Source: CAD feature listing. Evaluate the final solid. Frame: model axes, mm. Face numbers are marked on the shaded views. A direction names the side the tool comes from. Round coordinates to 2 decimals unless told otherwise and drop trailing zeros. Loops run counter-clockwise (first coordinate to the right, second up) from the corner with the lowest first, then second, coordinate; pieces in that order, holes last. Notation, with made-up numbers: M 76.25,-5 L 134.25,-5 A22 ccw 134.25,12 Z; hole C -33,-23 d4. An arc over 180 degrees is marked long. One line per item, written item: value.
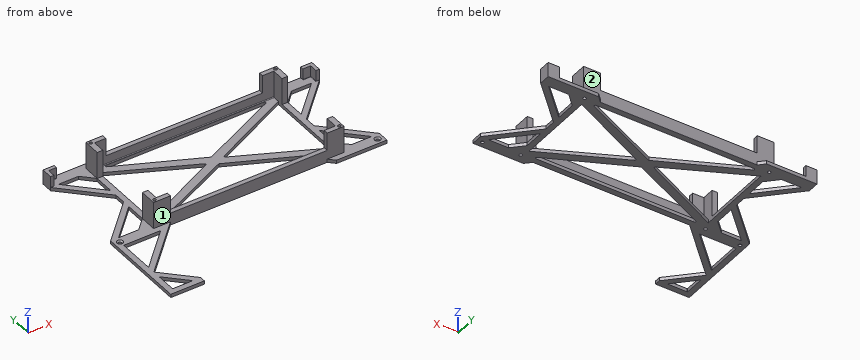
from build123d import *

# Parameters (mm, degrees)
SKETCH003_W     = 170
SKETCH003_H     = 90
SKETCH003_W_2   = 160
SKETCH003_H_2   = 80
PAD_DEPTH       = 3
PAD001_DEPTH    = 3
PAD002_DEPTH    = 3
PAD003_DEPTH    = 3
PAD004_DEPTH    = 3
PAD005_DEPTH    = 10
PAD006_DEPTH    = 10
PAD007_DEPTH    = 24
SKETCH014_R     = 1.65
HOLE_DEPTH      = 30
SKETCH015_R     = 1.325
HOLE001_DEPTH   = 30
SKETCH016_R     = 1.325
HOLE002_DEPTH   = 30
SKETCH017_R     = 1.325
HOLE003_DEPTH   = 30
FILLET_R        = 0.3
FILLET001_R     = 0.3
FILLET002_R     = 0.3
FILLET003_R     = 0.3
FILLET004_R     = 0.3
FILLET005_R     = 0.3
FILLET006_R     = 0.3
FILLET007_R     = 0.3
FILLET008_R     = 0.3
FILLET009_R     = 0.3
SKETCH018_W     = 3.707428
SKETCH018_H     = 3.707435
PAD008_DEPTH    = 27
SKETCH019_W     = 4.325348
SKETCH019_H     = 3.769226
PAD009_DEPTH    = 27
SKETCH020_W     = 4.473305
SKETCH020_H     = 4.349049
PAD010_DEPTH    = 27
SKETCH021_W     = 3.413819
SKETCH021_H     = 3.638272
PAD011_DEPTH    = 27
SKETCH023_R     = 1.4
POCKET_DEPTH    = 30
SKETCH024_R     = 1.4
POCKET001_DEPTH = 30
SKETCH025_R     = 1.4
POCKET002_DEPTH = 30
SKETCH026_R     = 1.4
POCKET003_DEPTH = 30
SKETCH027_R     = 1.5
POCKET004_DEPTH = 5
CHAMFER_SIZE    = 1.2
SKETCH028_W     = 10
SKETCH028_H     = 1
POCKET005_DEPTH = 24
SKETCH029_W     = 10
SKETCH029_H     = 1
POCKET006_DEPTH = 24
SKETCH030_W     = 10
SKETCH030_H     = 1
POCKET007_DEPTH = 24
PAD012_DEPTH    = 3
SKETCH032_W     = 140
SKETCH032_H     = 4
PAD013_DEPTH    = 8
FILLET010_R     = 0.7
FILLET011_R     = 1


with BuildPart() as part:
    # Sketch003 → Pad (new body)
    with BuildSketch(Plane.XY):
        Rectangle(SKETCH003_W, SKETCH003_H)
        Rectangle(SKETCH003_W_2, SKETCH003_H_2, mode=Mode.SUBTRACT)
    extrude(amount=PAD_DEPTH)

    # Sketch005 → Pad001 (join)
    with BuildSketch(Plane.XY):
        Polygon((-70, 45), (-75, 50), (-120, 50), (-120, 40), (-85, 5), (-85, 12), (-113, 40), (-95, 40), (-85, 30), (-85, 45), align=None)
    extrude(amount=PAD001_DEPTH)

    # Sketch007 → Pad002 (join)
    with BuildSketch(Plane.XY):
        Polygon((70, 45), (75, 50), (120, 50), (120, 40), (85, 5), (85, 12), (113, 40), (95, 40), (85, 30), (85, 45), align=None)
    extrude(amount=PAD002_DEPTH)

    # Sketch008 → Pad003 (join)
    with BuildSketch(Plane.XY):
        Polygon((70, -45), (75, -50), (120, -50), (120, -40), (85, -5), (85, -12), (113, -40), (95, -40), (85, -30), (85, -45), align=None)
    extrude(amount=PAD003_DEPTH)

    # Sketch009 → Pad004 (join)
    with BuildSketch(Plane.XY):
        Polygon((-70, -45), (-75, -50), (-115, -90), (-90, -115), (-90, -120), (-120, -120), (-120, -50), (-120, -40), (-85, -5), (-85, -12), (-113, -40), (-95, -40), (-85, -30), (-85, -45), align=None)
        Polygon((-115, -50), (-115, -83), (-82, -50), align=None, mode=Mode.SUBTRACT)
        Polygon((-115, -97), (-115, -115), (-97, -115), align=None, mode=Mode.SUBTRACT)
    extrude(amount=PAD004_DEPTH)

    # Sketch011 (on Face23 of Pad004) → Pad005 (join)
    with BuildSketch(Plane.XY.offset(3)):
        Polygon((-120, 50), (-120, 40), (-117, 40), (-117, 47), (-110, 47), (-110, 50), align=None)
    extrude(amount=PAD005_DEPTH)

    # Sketch012 (on Face22 of Pad005) → Pad006 (join)
    with BuildSketch(Plane.XY.offset(3)):
        Polygon((120, 50), (110, 50), (110, 47), (117, 47), (117, 40), (120, 40), align=None)
    extrude(amount=PAD006_DEPTH)

    # Sketch013 (on Face4 of Pad006) → Pad007 (join)
    with BuildSketch(Plane.XY.offset(3)):
        Polygon((-85, 45), (-85, 30), (-80, 30), (-80, 40), (-70, 40), (-70, 45), align=None)
        Polygon((85, 45), (85, 30), (80, 30), (80, 40), (70, 40), (70, 45), align=None)
        Polygon((85, -45), (85, -30), (80, -30), (80, -40), (70, -40), (70, -45), align=None)
        Polygon((-85, -45), (-85, -30), (-80, -30), (-80, -40), (-70, -40), (-70, -45), align=None)
    extrude(amount=PAD007_DEPTH)

    # Sketch014 (on Face80 of Pad007) → Hole (cut)
    with BuildSketch(Plane.XY.offset(27)):
        with Locations((-82.5, 42.5)):
            Circle(SKETCH014_R)
    extrude(amount=-HOLE_DEPTH, mode=Mode.SUBTRACT)

    # Sketch015 (on Face99 of Hole) → Hole001 (cut)
    with BuildSketch(Plane.XY.offset(27)):
        with Locations((-82.5, -42.5)):
            Circle(SKETCH015_R)
    extrude(amount=-HOLE001_DEPTH, mode=Mode.SUBTRACT)

    # Sketch016 (on Face84 of Hole001) → Hole002 (cut)
    with BuildSketch(Plane.XY.offset(27)):
        with Locations((82.5, 42.5)):
            Circle(SKETCH016_R)
    extrude(amount=-HOLE002_DEPTH, mode=Mode.SUBTRACT)

    # Sketch017 (on Face104 of Hole002) → Hole003 (cut)
    with BuildSketch(Plane.XY.offset(27)):
        with Locations((82.5, -42.5)):
            Circle(SKETCH017_R)
    extrude(amount=-HOLE003_DEPTH, mode=Mode.SUBTRACT)

    # Fillet
    fillet_edges = [part.edges().sort_by_distance(p)[0] for p in [
        (-115, -97, 1.5),
    ]]
    fillet(fillet_edges, radius=FILLET_R)

    # Fillet001
    fillet001_edges = [part.edges().sort_by_distance(p)[0] for p in [
        (-115, -115, 1.5),
    ]]
    fillet(fillet001_edges, radius=FILLET001_R)

    # Fillet002
    fillet002_edges = [part.edges().sort_by_distance(p)[0] for p in [
        (-97, -115, 1.5),
    ]]
    fillet(fillet002_edges, radius=FILLET002_R)

    # Fillet003
    fillet003_edges = [part.edges().sort_by_distance(p)[0] for p in [
        (-115, -90, 1.5),
    ]]
    fillet(fillet003_edges, radius=FILLET003_R)

    # Fillet004
    fillet004_edges = [part.edges().sort_by_distance(p)[0] for p in [
        (-115, -50, 1.5),
        (-115, -83, 1.5),
        (-82, -50, 1.5),
    ]]
    fillet(fillet004_edges, radius=FILLET004_R)

    # Fillet005
    fillet005_edges = [part.edges().sort_by_distance(p)[0] for p in [
        (-95, -40, 1.5),
        (-85, -12, 1.5),
        (-113, -40, 1.5),
    ]]
    fillet(fillet005_edges, radius=FILLET005_R)

    # Fillet006
    fillet006_edges = [part.edges().sort_by_distance(p)[0] for p in [
        (-117, 43.5, 3),
        (-113.5, 47, 3),
    ]]
    fillet(fillet006_edges, radius=FILLET006_R)

    # Fillet007
    fillet007_edges = [part.edges().sort_by_distance(p)[0] for p in [
        (-113, 40, 1.5),
        (-85, 12, 1.5),
    ]]
    fillet(fillet007_edges, radius=FILLET007_R)

    # Fillet008
    fillet008_edges = [part.edges().sort_by_distance(p)[0] for p in [
        (113.5, 47, 3),
        (117, 43.5, 3),
        (113, 40, 1.5),
        (85, 12, 1.5),
    ]]
    fillet(fillet008_edges, radius=FILLET008_R)

    # Fillet009
    fillet009_edges = [part.edges().sort_by_distance(p)[0] for p in [
        (113, -40, 1.5),
        (85, -12, 1.5),
    ]]
    fillet(fillet009_edges, radius=FILLET009_R)

    # Sketch018 (on Face81 of Fillet009) → Pad008 (join)
    with BuildSketch(Plane.XY.offset(27)):
        with Locations((82.542801, -42.437325)):
            Rectangle(SKETCH018_W, SKETCH018_H)
    extrude(amount=-PAD008_DEPTH)

    # Sketch019 (on Face37 of Pad008) → Pad009 (join)
    with BuildSketch(Plane.XY.offset(27)):
        with Locations((82.440964, 42.612553)):
            Rectangle(SKETCH019_W, SKETCH019_H)
    extrude(amount=-PAD009_DEPTH)

    # Sketch020 (on Face85 of Pad009) → Pad010 (join)
    with BuildSketch(Plane.XY.offset(27)):
        with Locations((-82.434589, 42.41842)):
            Rectangle(SKETCH020_W, SKETCH020_H)
    extrude(amount=-PAD010_DEPTH)

    # Sketch021 (on Face18 of Pad010) → Pad011 (join)
    with BuildSketch(Plane.XY.offset(27)):
        with Locations((-82.443809, -42.548483)):
            Rectangle(SKETCH021_W, SKETCH021_H)
    extrude(amount=-PAD011_DEPTH)

    # Sketch023 (on Face83 of Pad011) → Pocket (cut)
    with BuildSketch(Plane.XY.offset(27)):
        with Locations((-82.5, 42.5)):
            Circle(SKETCH023_R)
    extrude(amount=-POCKET_DEPTH, mode=Mode.SUBTRACT)

    # Sketch024 (on Face99 of Hole) → Pocket001 (cut)
    with BuildSketch(Plane.XY.offset(27)):
        with Locations((-82.5, -42.5)):
            Circle(SKETCH024_R)
    extrude(amount=-POCKET001_DEPTH, mode=Mode.SUBTRACT)

    # Sketch025 (on Face84 of Hole001) → Pocket002 (cut)
    with BuildSketch(Plane.XY.offset(27)):
        with Locations((82.5, 42.5)):
            Circle(SKETCH025_R)
    extrude(amount=-POCKET002_DEPTH, mode=Mode.SUBTRACT)

    # Sketch026 (on Face104 of Hole002) → Pocket003 (cut)
    with BuildSketch(Plane.XY.offset(27)):
        with Locations((82.5, -42.5)):
            Circle(SKETCH026_R)
    extrude(amount=-POCKET003_DEPTH, mode=Mode.SUBTRACT)

    # Sketch027 (on Face6 of Pocket003) → Pocket004 (cut)
    with BuildSketch(Plane.XY.offset(3)):
        with Locations((-115, -45)):
            Circle(SKETCH027_R)
        with Locations((115, -45)):
            Circle(SKETCH027_R)
    extrude(amount=-POCKET004_DEPTH, mode=Mode.SUBTRACT)

    # Chamfer
    chamfer_edges = [part.edges().sort_by_distance(p)[0] for p in [
        (-116.5, -45, 3),
        (113.5, -45, 3),
    ]]
    chamfer(chamfer_edges, length=CHAMFER_SIZE)

    # Sketch028 (on Face51 of Chamfer) → Pocket005 (cut)
    with BuildSketch(Plane.XY.offset(27)):
        with Locations((-75, 40.5)):
            Rectangle(SKETCH028_W, SKETCH028_H)
    extrude(amount=-POCKET005_DEPTH, mode=Mode.SUBTRACT)

    # Sketch029 (on Face96 of Pocket005) → Pocket006 (cut)
    with BuildSketch(Plane.XY.offset(27)):
        with Locations((75, 40.5)):
            Rectangle(SKETCH029_W, SKETCH029_H)
    extrude(amount=-POCKET006_DEPTH, mode=Mode.SUBTRACT)

    # Sketch030 (on Face98 of Pocket006) → Pocket007 (cut)
    with BuildSketch(Plane.XY.offset(27)):
        with Locations((75, -40.5)):
            Rectangle(SKETCH030_W, SKETCH030_H)
        with Locations((-75, -40.5)):
            Rectangle(SKETCH030_W, SKETCH030_H)
    extrude(amount=-POCKET007_DEPTH, mode=Mode.SUBTRACT)

    # Sketch031 → Pad012 (join)
    with BuildSketch(Plane.XY):
        Polygon((-80, 40), (-75, 40), (0, 5), (75, 40), (80, 40), (80, 35), (7, 0), (80, -35), (80, -40), (75, -40), (0, -5), (-75, -40), (-80, -40), (-80, -35), (-7, 0), (-80, 35), align=None)
    extrude(amount=PAD012_DEPTH)

    # Sketch032 (on Face109 of Pad012) → Pad013 (join)
    with BuildSketch(Plane.XY.offset(3)):
        with Locations((0, 43)):
            Rectangle(SKETCH032_W, SKETCH032_H)
        with Locations((0, -43)):
            Rectangle(SKETCH032_W, SKETCH032_H)
    extrude(amount=PAD013_DEPTH)

    # Fillet010
    fillet010_edges = [part.edges().sort_by_distance(p)[0] for p in [
        (0, 41, 3),
        (0, -41, 3),
    ]]
    fillet(fillet010_edges, radius=FILLET010_R)

    # Fillet011
    fillet011_edges = [part.edges().sort_by_distance(p)[0] for p in [
        (7, 0, 1.5),
        (-7, 0, 1.5),
        (-75, 40, 1.5),
        (-75, -40, 1.5),
        (75, -40, 1.5),
        (75, 40, 1.5),
    ]]
    fillet(fillet011_edges, radius=FILLET011_R)


solid = part.part
1. Reachability of the marked faces 1 and 2 from +Z, -Z, +X, -X, +Y, -Y: full face, straight path, thin tool, end or side. Return the list, or none.
Report:
face 1: +Z, -Y
face 2: +Z, +Y
2. Ray query, line 1 (Y direction, x = 115, z = 1.45); line 2 (Y direction, x = 82.5, z = 11); line 3 (Y direction, x = 45, z = 7). Return the intervals inside material, ascending. Write a range as [from, to].
Report:
line 1: y = [-50, -46.5], [-43.5, -35], [35, 50]
line 2: y = [-45, -43.9], [-41.1, -30], [30, 41.1], [43.9, 45]
line 3: y = [-45, -41], [41, 45]
3. Section query B-B (x = -49). Return the cut outline in (y, z), and give its area (3 significant figures).
Report:
outline: M -45,0 L -40,0 L -40,3 L -40.3,3 A0.7 cw -41,3.7 L -41,11 L -45,11 Z; M -27.87,0 L -20.14,0 L -20.14,3 L -27.87,3 Z; M 20.14,0 L 27.87,0 L 27.87,3 L 20.14,3 Z; M 40,0 L 45,0 L 45,11 L 41,11 L 41,3.7 A0.7 cw 40.3,3 L 40,3 Z
area: 141 mm2
4. Section query C-C (z = 8.5). Count the separate pieces of the cut face and the enclosed holes in it, and give its area (3 significant figures).
Report:
separate pieces: 4
enclosed holes: 4
area: 1,660 mm2
5. Pin query (flat end, axial travel): pin 1 (8 mm diameter, centred on y = -84.5, z = 6.5, fed in from +X); pin 2 (5 mm diameter, centred on x = 8.5, z = 11.5, fed in from -Y); pin 3 (3 mm diameter, centred on y = -31.5, z = 7, fed in from +X). Return the tip coordinate at first contact, or that it passes through.
Report:
pin 1: stops at x = -107.56
pin 2: stops at y = -45
pin 3: stops at x = 85
6. Section query A-A (z = 20.75). Return the cut outline in (x, y), and give its area (3 significant figures).
Report:
outline: M -85,-45 L -70,-45 L -70,-41 L -80,-41 L -80,-30 L -85,-30 Z; M -85,30 L -80,30 L -80,41 L -70,41 L -70,45 L -85,45 Z; M 70,-45 L 85,-45 L 85,-30 L 80,-30 L 80,-41 L 70,-41 Z; M 70,41 L 80,41 L 80,30 L 85,30 L 85,45 L 70,45 Z; hole C -82.5,-42.5 d2.8; hole C -82.5,42.5 d2.8; hole C 82.5,-42.5 d2.8; hole C 82.5,42.5 d2.8
area: 435 mm2
